Could you check a few things on this model? Use its own coordinates, in mm. A direction names the side the tool comes from. Coordinates: 2 decimals unless noted, no trailing zeros. Order: outer loops, then holes, each group sorted by start corner. A loop starts at its lowest first (then second) coordinate and runs counter-clockwise, first axis right, second up.
```python
from build123d import *

# Parameters (mm, degrees)
SKETCH11_W         = 98.552
SKETCH11_H         = 22.225
SKETCH11_R         = 3.19405
SKETCH11_R_2       = 4.76885
EXTRUDE3_DEPTH     = 7.9375
CUT_EXTRUDE1_DEPTH = 14.3002
FILLET1_R          = 6.35


with BuildPart() as part:
    # Sketch11 → Extrude3 (new body, symmetric)
    with BuildSketch(Plane.XY):
        with Locations((-42.926, 4.7625)):
            Rectangle(SKETCH11_W, SKETCH11_H)
        Circle(SKETCH11_R, mode=Mode.SUBTRACT)
        with Locations((-28.575, 3.175)):
            Circle(SKETCH11_R_2, mode=Mode.SUBTRACT)
    extrude(amount=EXTRUDE3_DEPTH, both=True)

    # Sketch12 → Cut-Extrude1 (cut)
    with BuildSketch(Plane.XZ.offset(6.35)):
        with BuildLine():
            Line((-7.9248, 4.0894), (6.35, 4.0894))
            Line((6.35, 4.0894), (6.35, -4.0894))
            Line((6.35, -4.0894), (-7.9248, -4.0894))
            ThreePointArc((-7.9248, -4.0894), (-12.0142, 0), (-7.9248, 4.0894))
        make_face()
    extrude(amount=-CUT_EXTRUDE1_DEPTH, mode=Mode.SUBTRACT)

    # Fillet1
    fillet1_edges = [part.edges().sort_by_distance(p)[0] for p in [
        (6.35, -6.35, -6.01345),
        (6.35, 15.875, 0),
        (6.35, -6.35, 6.01345),
    ]]
    fillet(fillet1_edges, radius=FILLET1_R)


solid = part.part
```
Item 1: Suppose I cut it at C-C (z = -3). List the corners of the cut face in (x, y) for me (3 decimals).
Item 2: Suppose I cut it at A-A (y = 6.5). List the corners of the cut face in (x, z) for me, and give its area (3 significant figures).
Item 3: I need wall thicknesses on line 1 (Y direction, x = 0, z = 5.4) (3 decimals); line 2 (X direction, y = 1, z = 5.25); line 3 (X direction, y = 10, z = 2.75). Which ranges of each line are inside material? Lowest first, please.
Item 4: Suppose I cut it at D-D (z = 7). List the corners of the cut face in (x, y) for me (3 decimals).
Item 5: Which directions (+Z, -Z, +X, -X, +Y, -Y) give clear straight access to the entire face, cutting with the end or side of a thin tool? Please do faces 1 (the face through (-24.026, 4.607, -0.111)), 2 (the face through (-12.013, 0.7, -0.09)).
Item 6: Thinking about a two-plate mould opening in X: for faces 3 (the face through (3.047, 0.959, 5.987)), 4 (the face through (-47, 15.875, 0)), 5 (the face through (6.35, 9, 0)), which applies, +X half, -X half, draft (parallel to the pull), parting line (faces both ways), or undercut?
Geometry results:
1. outline: (-92.202, -6.35) - (-10.704, -6.35) - (-10.704, 7.95) - (6.35, 7.95) - (6.35, 9.525) arc R6.35 ccw to (0, 15.875) - (-92.202, 15.875) - close; hole circle Ø9.538 at (-28.575, 3.175)
2. outline: (-92.2, -7.94) - (-31.99, -7.94) - (-31.99, 7.94) - (-92.2, 7.94) - close; (-25.16, -7.94) - (6.35, -7.94) - (6.35, -4.09) - (-7.92, -4.09) arc R4.09 cw to (-7.92, 4.09) - (6.35, 4.09) - (6.35, 7.94) - (-25.16, 7.94) - close
2. area: 1,310 mm2
3. line 1: y = -6.35 to -3.194, 3.194 to 15.875
3. line 2: x = -92.2 to -32.82, -24.33 to -3.03, 3.03 to 6.35
3. line 3: x = -92.2 to 6.33
4. outline: (-92.202, -6.35) - (0, -6.35) arc R6.35 ccw to (6.35, 0) - (6.35, 9.525) arc R6.35 ccw to (0, 15.875) - (-92.202, 15.875) - close; hole circle Ø9.538 at (-28.575, 3.175); hole circle Ø6.388 at (0, 0)
5. face 1: +Z, -Z
5. face 2: +X, -Y
6. face 3: undercut
6. face 4: draft
6. face 5: +X half
